Autodesk Inventor part; units mm, degrees
ref_plane "YZ Plane" through (0, 0, 0) normal (1, 0, 0) x (0, 1, 0)
ref_plane "XZ Plane" through (0, 0, 0) normal (0, 1, 0) x (-1, 0, 0)
ref_plane "XY Plane" through (0, 0, 0) normal (0, 0, 1) x (1, 0, 0)
sketch "草圖1" plane through (0, 0, 0) normal (0, 0, 1) x (1, 0, 0)
  line L0 (0, 0) -> (50, 0)
  line L1 (50, 0) -> (50, 40)
  line L2 (50, 40) -> (0, 40)
  line L3 (0, 40) -> (0, 0)
  dimension "d0" = 50
  dimension "d1" = 40
extrude "擠出1" add sketch "草圖1" along normal blind 40
sketch "草圖2" plane through (0, 40, 0) normal (0, 1, 0) x (1, 0, 0)
  line L0 (50, 0) -> (0, 0)
  line L1 (0, 0) -> (0, -40)
  line L2 (50, -40) -> (0, -40)
  line L3 (50, 0) -> (50, -40)
  line L4 (10, -40) -> (10, -20)
  line L5 (10, -20) -> (20, -10.2609)
  line L6 (20, -10.2609) -> (50, -10.2609)
  line L7 (50, 0) -> (50, -40)
  point P0 (0, 0)
  dimension "d4" = 10
  dimension "d5" = 10.2608
  dimension "d6" = 30
  dimension "d7" = 20
extrude "擠出2" cut sketch "草圖2" against normal blind 10 contours L3 L2 L4 L5 L6
sketch "草圖3" plane through (0, 30, 0) normal (0, 1, 0) x (1, 0, 0)
  line L0 (50, -10.2609) -> (50, -40)
  line L1 (20, -10.2609) -> (50, -10.2609)
  line L2 (10, -20) -> (20, -10.2609)
  line L3 (10, -40) -> (10, -20)
  line L4 (50, -40) -> (10, -40)
  line L5 (10, -29.7391) -> (30, -10.2609)
  point P0 (0, 0)
  dimension "d10" = 10
extrude "擠出3" cut sketch "草圖3" against normal blind 10 contours L0 L4 L3 L5 L1
sketch "草圖4" plane through (0, 20, 0) normal (0, 1, 0) x (1, 0, 0)
  line L0 (50, -10.2609) -> (50, -40)
  line L1 (30, -10.2609) -> (50, -10.2609)
  line L2 (10, -29.7391) -> (30, -10.2609)
  line L3 (10, -40) -> (10, -29.7391)
  line L4 (50, -40) -> (10, -40)
  line L5 (0, -40) -> (50, -40)
  line L6 (30, -20) -> (50, -40)
  line L7 (30, -20) -> (10, -40)
  point P0 (0, 0)
  dimension "d15" = 20
extrude "擠出4" cut sketch "草圖4" against normal blind 10 contours L4 L7 L6
Check sheet for the modelled part. Datum: model origin and axes. Units: mm. A direction names the side the tool comes from. Round coordinates to 2 decimals unless told otherwise and drop trailing zeros. Write each loop counter-clockwise with the first axis right and the second up, starting at its lowest first coordinate (ties: lowest second). Pieces come first, ordered by that corner, then holes. Notation, with made-up numbers: (-28.75, 71.5) -> (23.25, 71.5) arc R26 ccw to (23.25, 99.5) -> close; hole circle Ø4 at (-31.5, -30). An arc over 180 degrees is marked (long way). One line per question, with ' | ' between items. Start each with the question number.
1. Release check for a two-part mould opening along X. For faces 1 (the face through (20, 15, 30)), 2 (the face through (0, 20, 20)), 3 (the face through (14, 7, 40)) record: +X half, -X half, draft (parallel to the pull), parting line (faces both ways), or undercut.
2. Scan lines: line 1 along Y through (x, z) = (10.5, 24); line 2 along Y through (x, z) = (39, 11); line 3 along X through (y, z) = (16, 30.5). Record each from-to range of solid material in increasing order. Write a range as from..to.
3. Set-up check for faces 4 (the face through (34, 20, 22)), 5 (the face through (50, 15, 15)), 6 (the face through (30, 10, 32)): record each of +Z, -Z, +X, -X, +Y, -Y from which the full face is reachable in a straight line by a thin tool's end or side.
4. Sectioned sample at D-D, the plane y = 33.5. Record the cut outline in (x, z).
5. Depth check by flat-ended pin: pin 1 (10 mm diameter, centred on y = 26.5, z = 30.5, fed in from +X); pin 2 (2 mm diameter, centred on y = 11.5, z = 20.5, fed in from -X); pin 3 (4 mm diameter, centred on x = 18, z = 20, fed in from +Y); pin 4 (16 mm diameter, centred on x = 20.5, z = 33, fed in from +Y). Enter the tip coordinate at first touch or a pass-through.
6. Sectioned sample at A-A, the plane z = 36.5. Record the cut outline in (x, y).
7. Sectioned sample at B-B, the plane x = 42.5. Record the cut outline in (y, z), then the cut area to 3 significant figures.
8. Sectioned sample at C-C, the plane y = 24.5. Record the cut outline in (x, z), then the cut area to 3 significant figures.
Taken from the geometry:
1) face 1: undercut | face 2: -X half | face 3: draft
2) line 1: y = 0..30 | line 2: y = 0..20 | line 3: x = 0..19.5, 40.5..50
3) face 4: +Z, +X, +Y | face 5: +Z, -Z, +X, +Y, -Y | face 6: +Z, +Y
4) outline: (0, 0) -> (50, 0) -> (50, 10.26) -> (20, 10.26) -> (10, 20) -> (10, 40) -> (0, 40) -> close
5) pin 1: stops at x = 14.35 | pin 2: stops at x = 0 | pin 3: stops at y = 30 | pin 4: stops at y = 20
6) outline: (0, 0) -> (50, 0) -> (50, 20) -> (46.5, 20) -> (46.5, 10) -> (13.5, 10) -> (13.5, 20) -> (10, 20) -> (10, 40) -> (0, 40) -> close
7) outline: (0, 0) -> (40, 0) -> (40, 10.26) -> (20, 10.26) -> (20, 32.5) -> (10, 32.5) -> (10, 40) -> (0, 40) -> close | area: 930 mm^2
8) outline: (0, 0) -> (50, 0) -> (50, 10.26) -> (30, 10.26) -> (10, 29.74) -> (10, 40) -> (0, 40) -> close | area: 1,010 mm^2
